from build123d import *

# Parameters (mm, degrees)
F0_R     = 1.5875
F0_R_2   = 3.96875
F1_DEPTH = 19.05
F2_R     = 1.5875
F3_DEPTH = 52.578


with BuildPart() as f1:
    # F0 (on Right) → F1 (new body)
    with BuildSketch(Plane.YZ):
        with BuildLine():
            Line((414.526317, -10.552206), (414.526317, 17.834656))
            ThreePointArc((414.526317, 17.834656), (410.740304, 26.880696), (401.639572, 30.533283))
            Line((401.639572, 30.533283), (-436.560428, 18.206813))
            ThreePointArc((-436.560428, 18.206813), (-445.419722, 14.422173), (-449.073683, 5.508186))
            Line((-449.073683, 5.508186), (-449.073683, -10.552206))
            ThreePointArc((-449.073683, -10.552206), (-445.353939, -19.532462), (-436.373683, -23.252206))
            Line((-436.373683, -23.252206), (401.826317, -23.252206))
            ThreePointArc((401.826317, -23.252206), (410.806573, -19.532462), (414.526317, -10.552206))
        make_face()
        with Locations((-93.473683, 0)):
            Circle(F0_R, mode=Mode.SUBTRACT)
        with Locations((370.076317, 0)):
            Circle(F0_R_2, mode=Mode.SUBTRACT)
    extrude(amount=F1_DEPTH)

    # F2 (on face) → F3 (cut)
    with BuildSketch(Plane(origin=(0, 0, -23.252206), x_dir=(1, 0, 0), z_dir=(0, 0, -1))):
        with Locations((9.525, -668.526317)):
            Circle(F2_R)
    extrude(amount=-F3_DEPTH, mode=Mode.SUBTRACT)


solid = f1.part
Here's how the part is built. I have some questions about the finished solid (model axes, mm). Round coordinates to 2 decimals unless told otherwise and drop trailing zeros. Order: outer loops, then holes, each group sorted by start corner. A loop starts at its lowest first (then second) coordinate and runs counter-clockwise, first axis right, second up. Notation, with made-up numbers: (-3, 4.25) -> (33, 4.25) arc R30 cw to (33, 32.25) -> close; hole circle Ø8 at (73, -10.5). An arc over 180 degrees is marked (long way). Return JSON: item names as keys, results as strings.
Q1. For pin 1 Ø3 at (x, y) = (17, 258) entering from +Z; pin 2 Ø6 at (x, y) = (7, -269) entering from +Z; pin 3 Ø1 at (x, z) = (8, 13.5) entering from -Y; pin 4 Ø7 at (y, z) = (370.08, 0) entering from -X, each with a flat end and sliding along its axis, tell me the tip position at first contact or that it passes through.
Filled sheet:
{"pin 1": "stops at z = 28.44", "pin 2": "stops at z = 20.72", "pin 3": "stops at y = -446.63", "pin 4": "passes through"}
Q2. I need wall thicknesses on line 1 along Y through (x, z) = (16.5, -1); line 2 along Y through (x, z) = (12, 11); line 3 along Z through (x, y) = (7.75, 214). Which ranges of each line are inside material? Lowest first, please. Write a range as from..to.
Filled sheet:
{"line 1": "y = -449.07..-94.71, -92.24..366.24, 373.92..414.53", "line 2": "y = -447.82..414.53", "line 3": "z = -23.25..27.77"}
Q3. If we section it at A-A on x = 4.25: List the corners of the cut face in (y, z) for me (1 decimal).
Filled sheet:
{"outline": "(-449.1, -10.6) arc R12.7 ccw to (-436.4, -23.3) -> (401.8, -23.3) arc R12.7 ccw to (414.5, -10.6) -> (414.5, 17.8) arc R12.7 ccw to (401.6, 30.5) -> (-436.6, 18.2) arc R12.7 ccw to (-449.1, 5.5) -> close; hole circle Ø3.2 at (-93.5, 0); hole circle Ø7.9 at (370.1, 0)"}
Q4. If we section it at C-C on y = 245: List the corners of the cut face in (x, z) for me.
Filled sheet:
{"outline": "(0, -23.25) -> (19.05, -23.25) -> (19.05, 28.23) -> (0, 28.23) -> close"}
Q5. If we section it at B-B on y = 76.5: List the corners of the cut face in (x, z) for me, plus the area to 3 significant figures.
Filled sheet:
{"outline": "(0, -23.25) -> (19.05, -23.25) -> (19.05, 25.75) -> (0, 25.75) -> close", "area": "934 mm^2"}
